from build123d import *

# Parameters (mm, degrees)
SKETCH_1_R          = 100
EXTRUDE_1_DEPTH     = 20
SKETCH_2_R          = 1.5
CUT_EXTRUDE_1_DEPTH = 20


with BuildPart() as part:
    # 草图1 → 凸台-拉伸1 (new body)
    with BuildSketch(Plane.XY):
        Circle(SKETCH_1_R)
    extrude(amount=EXTRUDE_1_DEPTH)

    # 草图2 → 切除-拉伸1 (cut)
    with BuildSketch(Plane.XY.offset(20)):
        with Locations((0, 15.5)):
            Circle(SKETCH_2_R)
        with Locations((-15.5, 0)):
            Circle(SKETCH_2_R)
        with Locations((15.5, 0)):
            Circle(SKETCH_2_R)
        with Locations((0, -15.5)):
            Circle(SKETCH_2_R)
    extrude(amount=-CUT_EXTRUDE_1_DEPTH, mode=Mode.SUBTRACT)


solid = part.part
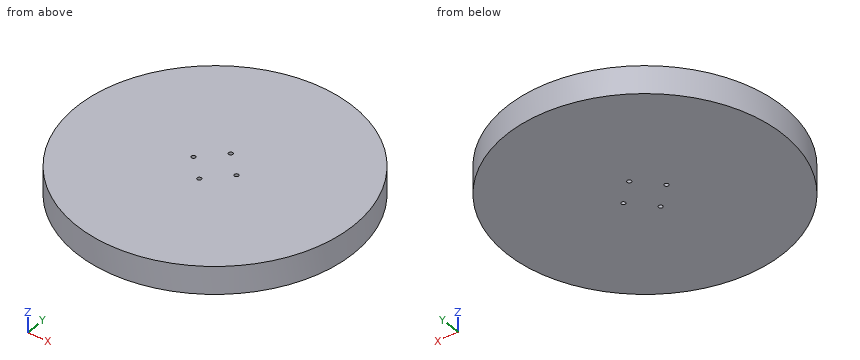
Build history of the part. All positions in model axes, mm. Round coordinates to 2 decimals unless told otherwise and drop trailing zeros. Loops run counter-clockwise (first coordinate to the right, second up) from the corner with the lowest first, then second, coordinate; pieces in that order, holes last. Notation, with made-up numbers: (54, -11.5) -> (63, -11.5) arc R20 cw to (63, 2.5) -> close; hole circle Ø11 at (48, -35.5). An arc over 180 degrees is marked (long way). One line per item, written item: value. Start each with the question number.
Q1. Cut at A-A on z = 3.25. List the corners of the cut face in (x, y), plus the area to 3 significant figures.
Q2. Probe line 1 along Y through (x, z) = (15.5, 12.75); line 2 along Y through (x, z) = (71, 7.25); line 3 along Y through (x, z) = (-18, 17.5). List the from-to ranges inside material, lowest first.
Q3. Cut at B-B on y = -60. List the corners of the cut face in (x, z), plus the area to 3 significant figures.
Q4. Cut at C-C on x = 42. List the corners of the cut face in (y, z).
Q5. Drop flat-ended pins along their axis: pin 1 Ø1 at (x, y) = (-75.5, -24.5) entering from -Z; pin 2 Ø2.5 at (x, y) = (-15.5, 0) entering from -Z; pin 3 Ø1.5 at (x, z) = (-48.5, 17.5) entering from +Y; pin 4 Ø12 at (y, z) = (62.5, 9) entering from -X. Give the stop position or say it passes through.
Computed:
1. outline: circle Ø200 at (0, 0); hole circle Ø3 at (-15.5, 0); hole circle Ø3 at (0, -15.5); hole circle Ø3 at (0, 15.5); hole circle Ø3 at (15.5, 0)
1. area: 31,400 mm²
2. line 1: -98.79 to -1.5, 1.5 to 98.79
2. line 2: -70.42 to 70.42
2. line 3: -98.37 to 98.37
3. outline: (-80, 0) -> (80, 0) -> (80, 20) -> (-80, 20) -> close
3. area: 3,200 mm²
4. outline: (-90.75, 0) -> (90.75, 0) -> (90.75, 20) -> (-90.75, 20) -> close
5. pin 1: z = 0
5. pin 2: through
5. pin 3: y = 87.86
5. pin 4: x = -82.51
